Design review of the part built by this model. Coordinates are the model's own, in mm. Round coordinates to 2 decimals unless told otherwise and drop trailing zeros. Order: outer loops, then holes, each group sorted by start corner. A loop starts at its lowest first (then second) coordinate and runs counter-clockwise, first axis right, second up. Notation, with made-up numbers: (-14, -3) - (42, -3) arc R21 cw to (42, 19) - close; hole circle Ø5 at (-7, -5.5). An arc over 180 degrees is marked (long way). Write item = value, one per line.
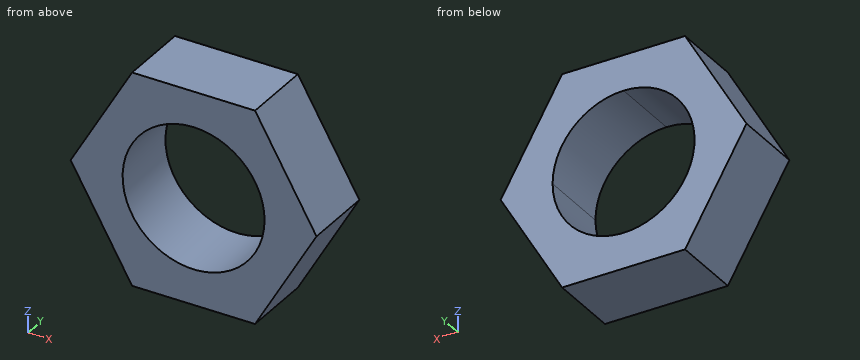
from build123d import *

# Parameters (mm, degrees)
F1_DEPTH = 12.7


with BuildPart() as f1:
    # F0 (on Front) → F1 (new body)
    with BuildSketch(Plane.XZ):
        Polygon((10.998523, 19.05), (0, 19.05), (-10.998523, 19.05), (-21.997045, 0), (-10.998523, -19.05), (10.998523, -19.05), (21.997045, 0), align=None)
        with BuildLine():
            ThreePointArc((12.7, 0), (-8.980256, -8.980256), (0, 12.7))
            ThreePointArc((0, 12.7), (8.980256, 8.980256), (12.7, 0))
        make_face(mode=Mode.SUBTRACT)
    extrude(amount=F1_DEPTH)


solid = f1.part
1) We need section D-D on z = -16. Write out the cut boundary in (x, y), and give its area (3 significant figures).
Findings:
outline = (-12.76, -12.7) - (12.76, -12.7) - (12.76, 0) - (-12.76, 0) - close
area = 324 mm^2
2) We need section B-B on x = 2. Write out the cut boundary in (y, z), and give its area (3 significant figures).
Findings:
outline = (-12.7, -19.05) - (0, -19.05) - (0, -12.54) - (-12.7, -12.54) - close; (-12.7, 12.54) - (0, 12.54) - (0, 19.05) - (-12.7, 19.05) - close
area = 165 mm^2
3) We need section C-C on y = -5. Write out the cut boundary in (x, z).
Findings:
outline = (-22, 0) - (-11, -19.05) - (11, -19.05) - (22, 0) - (11, 19.05) - (-11, 19.05) - close; hole circle Ø25.4 at (0, 0)
4) To check wall thickness, follow L1, parallel to Z at x = 0, y = -4.25; L2, parallel to X at y = -8.25, z = 6; L3, parallel to Z at x = -5.5, y = -1.25. State the ranges of each line that lie inside material, in increasing order. Write a range as from..to.
Findings:
L1 = -19.05..-12.7, 12.7..19.05
L2 = -18.53..-11.19, 11.19..18.53
L3 = -19.05..-11.45, 11.45..19.05
5) We need section A-A on z = 8. Write out the cut boundary in (x, y), and give its area (3 significant figures).
Findings:
outline = (-17.38, -12.7) - (-9.86, -12.7) - (-9.86, 0) - (-17.38, 0) - close; (9.86, -12.7) - (17.38, -12.7) - (17.38, 0) - (9.86, 0) - close
area = 191 mm^2
6) Clearance check with flat-ended pins moving along their axes: pin 1 Ø1 at (y, z) = (-5, 13.5) entering from -X; pin 2 Ø2 at (y, z) = (-8, -10) entering from +X; pin 3 Ø4 at (y, z) = (-6, -14) entering from +X. State where each tip first meets the part, or that it passes through.
Findings:
pin_1 = -14.49
pin_2 = 16.8
pin_3 = 15.07
